Autodesk Fusion 360 part; units mm, degrees
sketch "Sketch1" plane through (0, 0, 0) normal (0, 1, 0) x (1, 0, 0)
  line L0 (33, 21) -> (-33, 21)
  line L1 (-33, 21) -> (-33, -21)
  line L2 (-33, -21) -> (33, -21)
  line L3 (33, -21) -> (33, 21)
  line L4 (33, 21) -> (-33, -21) construction
  line L5 (-33, 21) -> (33, -21) construction
  dimension "d1" = 66
extrude "Extrude1" add sketch "Sketch1" along normal blind 12
chamfer "Chamfer1" distance 12 angle 45 2 edges at (33, 6, 21) (33, 6, -21)
sketch "Sketch2" plane through (0, 12, 0) normal (0, 1, 0) x (-1, 0, 0)
  line L0 (-33, -9) -> (-21, -21)
  line L1 (-21, -21) -> (33, -21)
  line L2 (33, -21) -> (33, 21)
  line L3 (33, 21) -> (-21, 21)
  line L4 (-21, 21) -> (-33, 9)
  line L5 (-33, 9) -> (-33, -9)
  line L6 (33, 21) -> (21, 21)
  line L7 (21, 21) -> (21, -21)
  line L8 (21, -21) -> (33, -21)
  line L9 (33, -21) -> (33, 21)
  dimension "d6" = 12
extrude "Extrude2" add sketch "Sketch2" along normal blind 48 contours L1 L2 L3 L6 L7 L8 L9
fillet "Fillet1" radius 21 2 edges at (-27, 60, 21) (-27, 60, -21)
sketch "Sketch3" plane through (0, 0, 0) normal (0, 1, 0) x (1, 0, 0)
sketch "Sketch4" plane through (0, 0, 0) normal (0, 0, 1) x (1, 0, 0)
  line L0 (-21.0139, 54) -> (-21.0139, 12)
  line L1 (-21.0139, 12) -> (32.9285, 12)
  line L2 (32.9285, 12) -> (-21.0139, 54)
  dimension "d11" = 42
extrude "Extrude3" add sketch "Sketch4" along normal blind 6
extrude "Extrude4" add 1 faces at (-3.0238, 25.9964, 0) along direction (0, 0, -1) mid plane 12
sketch "Sketch5" plane through (0, 0, 0) normal (1, 0, 0) x (0, 0, -1)
equation "d7 = 60 mm - 12 mm"
For this review, take the finished solid that the model builds, in its own axes (mm). A direction names the side the tool comes from. Round coordinates to 2 decimals unless told otherwise and drop trailing zeros. Write each loop counter-clockwise with the first axis right and the second up, starting at its lowest first coordinate (ties: lowest second). Pieces come first, ordered by that corner, then holes. Notation, with made-up numbers: (66.25, 86.5) -> (83.25, 86.5) arc R7 cw to (83.25, 96.5) -> close; hole circle Ø3 at (-25, 82). An arc over 180 degrees is marked (long way). One line per question, with ' | ' between items. Start each with the question number.
1) Machinability: for faces 1 (the flat face through (6.34, 32.7, -0.08)), 2 (the flat face through (-21, 36, 10)), 3 (the flat face through (-6, 24, 6)), 4 (the flat face through (-6, 24, -6)), which of the approach directions +Z, -Z, +X, -X, +Y, -Y give a long, thin tool a straight path to every point of the face, cutting with its end or side? Answer none if there is none.
2) For pin 1 Ø21 at (y, z) = (45, 0.5) entering from +X; pin 2 Ø21 at (x, y) = (4.5, 30.5) entering from +Z; pin 3 Ø3 at (x, y) = (5.5, 22.5) entering from -Z; pin 4 Ø10 at (x, z) = (5.5, -14) entering from -Y, all flat-tipped, find the tip position at first contact; note any pin that passes through.
3) Add section D-D (z = 10.5). Write out the cut boundary in (x, y).
4) Add section A-A (x = 8). Write out the cut boundary in (y, z).
5) Wall thickness on line 1 along X through (y, z) = (31, -11); line 2 along Y through (x, z) = (-15, 10); line 3 along Z through (x, y) = (-2.5, 13.5): over which ranges is each line inside the solid? List them lowest first.
6) Add section B-B (z = -2). Write out the cut boundary in (x, y), and give its area (3 significant figures).
7) Add section C-C (y = 25.5). Write out the cut boundary in (x, z).
Reported:
1) face 1: +Z, -Z, +X, +Y | face 2: +X, +Y | face 3: +Z, +X, +Y | face 4: -Z, +X, +Y
2) pin 1: stops at x = 4.03 | pin 2: stops at z = 6 | pin 3: stops at z = -6 | pin 4: stops at y = 0
3) outline: (-33, 0) -> (31.5, 0) -> (31.5, 12) -> (-21, 12) -> (-21, 57.19) -> (-33, 57.19) -> close
4) outline: (0, -21) -> (12, -21) -> (12, -6) -> (31.41, -6) -> (31.41, 6) -> (12, 6) -> (12, 21) -> (0, 21) -> close
5) line 1: x = -33 to -21 | line 2: y = 0 to 12 | line 3: z = -6 to 6
6) outline: (-33, 0) -> (33, 0) -> (33, 12) -> (32.93, 12) -> (-21, 53.99) -> (-21, 59.9) -> (-33, 59.9) -> close | area: 2,500 mm²
7) outline: (-33, -21) -> (-21, -21) -> (-21, -6) -> (15.59, -6) -> (15.59, 6) -> (-21, 6) -> (-21, 21) -> (-33, 21) -> close
